Geometry: final body of the model. Coordinates: model frame, mm. Face numbers are marked on the shaded views. A direction names the side the tool comes from. Give positions to 0.01 mm unless a question says otherwise; leave off trailing zeros. Write each loop counter-clockwise with the first axis right and the second up, starting at its lowest first coordinate (ties: lowest second). Pieces come first, ordered by that corner, then holes.
from build123d import *

# Parameters (mm, degrees)
SKETCH1_R           = 1.6
BOSS_EXTRUDE1_DEPTH = 2
SKETCH2_W           = 96
SKETCH2_H           = 45
SKETCH2_W_2         = 92
SKETCH2_H_2         = 41
BOSS_EXTRUDE2_DEPTH = 10
SKETCH3_W           = 92
SKETCH3_H           = 41
CUT_EXTRUDE1_DEPTH  = 65.855608855
SKETCH4_W           = 96
SKETCH4_H           = 45
BOSS_EXTRUDE3_DEPTH = 2
CUT_EXTRUDE2_DEPTH  = 66.193941436
SKETCH6_W           = 30
SKETCH6_H           = 8
CUT_EXTRUDE4_DEPTH  = 66.193941436


with BuildPart() as part:
    # Sketch1 → Boss-Extrude1 (new body)
    with BuildSketch(Plane(origin=(0, 0, 0), x_dir=(1, 0, 0), z_dir=(0, 1, 0))):
        with BuildLine():
            Line((-48, 5), (-55, 5))
            ThreePointArc((-55, 5), (-60, 0), (-55, -5))
            Line((-55, -5), (-48, -5))
            Line((-48, -5), (-48, -22.5))
            Line((-48, -22.5), (48, -22.5))
            Line((48, -22.5), (48, -5))
            Line((48, -5), (55, -5))
            ThreePointArc((55, -5), (60, 0), (55, 5))
            Line((55, 5), (48, 5))
            Line((48, 5), (48, 22.5))
            Line((48, 22.5), (-48, 22.5))
            Line((-48, 22.5), (-48, 5))
        make_face()
        with Locations(Location((-55, 0, 0), (0, 0, 270))):
            Circle(SKETCH1_R, mode=Mode.SUBTRACT)
        with Locations(Location((55, 0, 0), (0, 0, 270))):
            Circle(SKETCH1_R, mode=Mode.SUBTRACT)
    extrude(amount=BOSS_EXTRUDE1_DEPTH)

    # Sketch2 → Boss-Extrude2 (add)
    with BuildSketch(Plane(origin=(0, 2, 0), x_dir=(1, 0, 0), z_dir=(0, 1, 0))):
        Rectangle(SKETCH2_W, SKETCH2_H)
        Rectangle(SKETCH2_W_2, SKETCH2_H_2, mode=Mode.SUBTRACT)
    extrude(amount=BOSS_EXTRUDE2_DEPTH)

    # Sketch3 → Cut-Extrude1 (cut, through all)
    with BuildSketch(Plane(origin=(0, 2, 0), x_dir=(1, 0, 0), z_dir=(0, 1, 0))):
        Rectangle(SKETCH3_W, SKETCH3_H)
    extrude(amount=-CUT_EXTRUDE1_DEPTH, mode=Mode.SUBTRACT)

    # Sketch4 → Boss-Extrude3 (add)
    with BuildSketch(Plane(origin=(0, 12, 0), x_dir=(1, 0, 0), z_dir=(0, 1, 0))):
        Rectangle(SKETCH4_W, SKETCH4_H)
    extrude(amount=BOSS_EXTRUDE3_DEPTH)

    # Sketch5 → Cut-Extrude2 (cut, through all)
    with BuildSketch(Plane(origin=(0, 12, 0), x_dir=(-1, 0, 0), z_dir=(0, -1, 0))):
        with BuildLine():
            ThreePointArc((42.6, -16), (42.13137085, -14.86862915), (41, -14.4))
            Line((41, -14.4), (41, -16))
            Line((41, -16), (39.4, -16))
            ThreePointArc((39.4, -16), (41, -17.6), (42.6, -16))
        make_face()
        with BuildLine():
            Line((41, -16), (41, -14.4))
            ThreePointArc((41, -14.4), (39.86862915, -14.86862915), (39.4, -16))
            Line((39.4, -16), (41, -16))
        make_face()
        with BuildLine():
            ThreePointArc((42.6, 16), (41, 17.6), (39.4, 16))
            Line((39.4, 16), (41, 16))
            Line((41, 16), (41, 14.4))
            ThreePointArc((41, 14.4), (42.13137085, 14.86862915), (42.6, 16))
        make_face()
        with BuildLine():
            Line((41, 16), (39.4, 16))
            ThreePointArc((39.4, 16), (39.86862915, 14.86862915), (41, 14.4))
            Line((41, 14.4), (41, 16))
        make_face()
        with BuildLine():
            ThreePointArc((-41, 14.4), (-39.86862915, 14.86862915), (-39.4, 16))
            Line((-39.4, 16), (-41, 16))
            Line((-41, 16), (-41, 14.4))
        make_face()
        with BuildLine():
            Line((-41, 16), (-39.4, 16))
            ThreePointArc((-39.4, 16), (-42.13137085, 17.13137085), (-41, 14.4))
            Line((-41, 14.4), (-41, 16))
        make_face()
        with BuildLine():
            ThreePointArc((-39.4, -16), (-39.86862915, -14.86862915), (-41, -14.4))
            Line((-41, -14.4), (-41, -16))
            Line((-41, -16), (-39.4, -16))
        make_face()
        with BuildLine():
            Line((-41, -16), (-41, -14.4))
            ThreePointArc((-41, -14.4), (-42.13137085, -17.13137085), (-39.4, -16))
            Line((-39.4, -16), (-41, -16))
        make_face()
    extrude(amount=-CUT_EXTRUDE2_DEPTH, mode=Mode.SUBTRACT)

    # Sketch6 → Cut-Extrude4 (cut, through all)
    with BuildSketch(Plane(origin=(0, 12, 0), x_dir=(-1, 0, 0), z_dir=(0, -1, 0))):
        with Locations((0, -16.5)):
            Rectangle(SKETCH6_W, SKETCH6_H)
    extrude(amount=-CUT_EXTRUDE4_DEPTH, mode=Mode.SUBTRACT)


solid = part.part
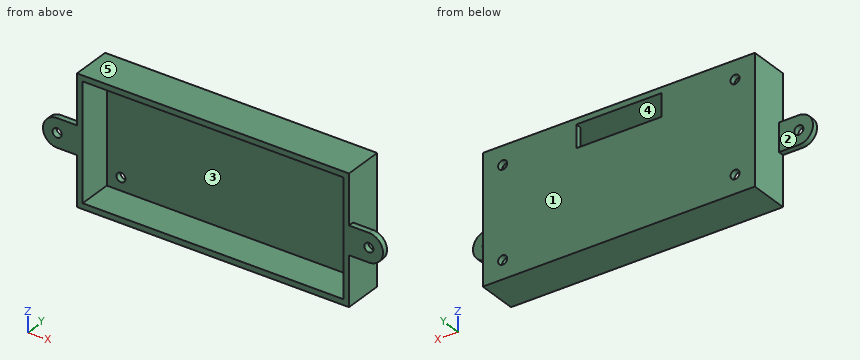
Q1. Ray query, line 1 along X through (y, z) = (12.6, 16); line 2 along Z through (x, y) = (41, 12.7); line 3 along Z through (x, y) = (-21.5, 11.5). Return the intervals inside material, ascending.
Filled sheet:
line 1: x = -48 to -42.6, -39.4 to -15, 15 to 39.4, 42.6 to 48
line 2: z = -22.5 to -17.6, -14.4 to 14.4, 17.6 to 22.5
line 3: z = -22.5 to -20.5, 20.5 to 22.5
Q2. Section D-D on z = -10.5. Output: boundary loops of the cut face in (x, y), plus the area to 3 significant figures.
Filled sheet:
outline: (-48, 0) - (-46, 0) - (-46, 12) - (46, 12) - (46, 0) - (48, 0) - (48, 14) - (-48, 14) - close
area: 240 mm2
Q3. Access query for the marked faces 1, 2 and 3. Directions: +Z, -Z, +X, -X, +Y, -Y. A direction counts if a zero-diameter tool reaches every point of the face in a straight line with its end or side. Return the directions, or none.
Filled sheet:
face 1: +Z, -Z, +X, -X, +Y
face 2: +Z, -Z, -X, +Y
face 3: -Y
Q4. Section A-A on y = 8.25. Output: boundary loops of the cut face in (x, z).
Filled sheet:
outline: (-48, -22.5) - (48, -22.5) - (48, 22.5) - (-48, 22.5) - close; hole (-46, -20.5) - (46, -20.5) - (46, 20.5) - (-46, 20.5) - close
Q5. Pin query (flat end, axial travel): P1, Ø8, axis at x = -56.5, z = 1.5, coming from the +Y side; P2, Ø1, axis at y = 3, z = 6, coming from the -X side; P3, Ø20.5, axis at x = 17, z = 5, coming from the -Y side. Return the tip coordinate at first contact, or that it passes through.
Filled sheet:
P1: stops at y = 2
P2: stops at x = -48
P3: stops at y = 12
Q6. Pull-direction query (X, two-part tool) for the marked faces 4 and 5; classes: released by +X, released by -X, zero draft, split by the parting line, or undercut.
Filled sheet:
face 4: undercut
face 5: zero draft
Q7. Section B-B on z = 0. Output: boundary loops of the cut face in (x, y).
Filled sheet:
outline: (-60, 0) - (-56.6, 0) - (-56.6, 2) - (-60, 2) - close; (-53.4, 0) - (-46, 0) - (-46, 12) - (46, 12) - (46, 0) - (53.4, 0) - (53.4, 2) - (48, 2) - (48, 14) - (-48, 14) - (-48, 2) - (-53.4, 2) - close; (56.6, 0) - (60, 0) - (60, 2) - (56.6, 2) - close
Q8. Section C-C on x = -1. Output: boundary loops of the cut face in (y, z), plus the area to 3 significant figures.
Filled sheet:
outline: (0, -22.5) - (14, -22.5) - (14, 12.5) - (12, 12.5) - (12, -20.5) - (0, -20.5) - close; (0, 20.5) - (14, 20.5) - (14, 22.5) - (0, 22.5) - close
area: 122 mm2
